Autodesk Inventor part; units mm, degrees
ref_plane "YZ Plane" through (0, 0, 0) normal (1, 0, 0) x (0, 1, 0)
ref_plane "XZ Plane" through (0, 0, 0) normal (0, 1, 0) x (-1, 0, 0)
ref_plane "XY Plane" through (0, 0, 0) normal (0, 0, 1) x (1, 0, 0)
sketch "Sketch1" plane through (0, 0, 0) normal (0, 0, 1) x (1, 0, 0)
  line L0 (0, 12.7112) -> (0, -15.7964)
  line L1 (-14.6857, 0) -> (16.9071, 0)
  line L2 (8.8388, 8.8388) -> (88.8388, -71.1612)
  line L3 (-8.8388, 8.8388) -> (-88.8388, -71.1612)
  line L4 (8.8388, -26.5165) -> (71.1612, -88.8388)
  line L5 (-8.8388, -26.5165) -> (-71.1612, -88.8388)
  arc A0 (8.8388, 8.8388) -> (-8.8388, 8.8388) centre (0, 0) ccw
  arc A1 (8.8388, -26.5165) -> (-8.8388, -26.5165) centre (0, -35.3553) ccw
  arc A2 (71.1612, -88.8388) -> (88.8388, -71.1612) centre (80, -80) ccw
  arc A3 (-88.8388, -71.1612) -> (-71.1612, -88.8388) centre (-80, -80) ccw
  circle A4 centre (-80, -80) radius 3.5
  circle A5 centre (80, -80) radius 3.5
  circle A6 centre (0, 0) radius 8.5
  point P0 (0, 17.6777)
  point P1 (0, -17.6777)
  dimension "d0" = 25
  dimension "d1" = 12.5
  dimension "d2" = 0
  dimension "d3" = 90
  dimension "d4" = 7
  dimension "d5" = 7
  dimension "d8" = 17
  dimension "d17" = 80
extrude "Extrusion1" add sketch "Sketch1" along normal blind 3
sketch "Sketch2" plane through (0, 0, 3) normal (0, 0, 1) x (1, 0, 0)
  circle A0 centre (80, -80) radius 3.5
  line L0 (80, -80) -> (55.28, -55.28)
  line L1 (88.8388, -71.1612) -> (8.8388, 8.8388)
  circle A1 centre (72.0098, -59.6354) radius 1.55
  circle A2 centre (59.6354, -72.0098) radius 1.55
  point P0 (0, 0)
  dimension "d9" = 3.1
  dimension "d10" = 3.1
  dimension "d11" = 21.876
  dimension "d12" = 17.5
extrude "Extrusion2" add sketch "Sketch2" along normal blind 10 contours A1 | A2
mirror "Mirror1" about plane through (0, 0, 0) normal (1, 0, 0) of "Extrusion2"
fillet "Fillet1" radius 2 4 edges at (-70.4598, -59.6354, 3) (-58.0854, -72.0098, 3) (70.4598, -59.6354, 3) (58.0854, -72.0098, 3)
properties part number "rockerbogieçükü"
Check sheet for the modelled part. Datum: model origin and axes. Units: mm. A direction names the side the tool comes from. Round coordinates to 2 decimals unless told otherwise and drop trailing zeros. Loops run counter-clockwise (first coordinate to the right, second up) from the corner with the lowest first, then second, coordinate; pieces in that order, holes last. Notation, with made-up numbers: M 68,-21.5 L 76,-21.5 A29 ccw 76,7.5 Z; hole C 20,27 d7. An arc over 180 degrees is marked long. Answer as a JSON object with one key per item and string values.
1. Section check D-D (y = -13). Record the boundary of the cut face in (x, z).
Reply:
{"outline": "M -30.68,0 L 30.68,0 L 30.68,3 L -30.68,3 Z"}
2. Section check B-B (x = 0). Record the boundary of the cut face in (y, z).
Reply:
{"outline": "M -22.86,0 L -8.5,0 L -8.5,3 L -22.86,3 Z; M 8.5,0 L 12.5,0 L 12.5,3 L 8.5,3 Z"}
3. Access from +Z, -Z, +X, -X, +Y, -Y to the whole of each face (thin tool, end or side, straight path). Record for faces 5 (the flat face through (-39.56, -57.24, 1.48)), 6 (the cylindrical face through (81.615, -76.895, 1.479)).
Reply:
{"face 5": "+Z, -Z, -Y", "face 6": "+Z, -Z"}
4. Scan lines: line 1 (Z direction, x = 13, y = 1); line 2 (Y direction, x = -80, z = 2.25); line 3 (X direction, y = 0, z = 1.55). Record each from-to range of solid material in increasing order.
Reply:
{"line 1": "z = 0 to 3", "line 2": "y = -92.5 to -83.5, -76.5 to -62.32", "line 3": "x = -17.68 to -8.5, 8.5 to 17.68"}
5. Mould release check, pull along Y, two halves, no side actions. Record for faces 1 (the cylindrical face through (4.57, -7.167, 1.479)), 2 (the flat face through (39.56, -57.24, 1.48)), 3 (the cylindrical face through (-78.385, -76.895, 1.479)), 4 (the flat face through (-14, -28, 0)): pulls with the +Y half, pulls with the -Y half, needs draft (parallel to the pull), parting line crosses it, or undercut.
Reply:
{"face 1": "undercut", "face 2": "pulls with the -Y half", "face 3": "undercut", "face 4": "needs draft"}
6. Gauge pin test, flat ends, axial feed: P1, Ø2, axis at x = 13.5, z = 1.5, coming from the +Y side; P2, Ø4, axis at x = -80, y = -80, coming from the -Z side; P3, Ø12, axis at x = -13.5, y = -4, coming from the +Z side; P4, Ø4, axis at y = -1, z = 4.5, coming from the +X side. Record the tip position at first contact, or that the pin passes through.
Reply:
{"P1": "stops at y = 5.18", "P2": "passes through", "P3": "stops at z = 3", "P4": "stops at x = 20"}
7. Section check A-A (y = -35.5). Record the boundary of the cut face in (x, z).
Reply:
{"outline": "M -53.18,0 L -17.82,0 L -17.82,3 L -53.18,3 Z; M 17.82,0 L 53.18,0 L 53.18,3 L 17.82,3 Z"}
8. Section check C-C (z = 8.75). Record the boundary of the cut face in (x, y), plus the area to 3 significant figures.
Reply:
{"outline": "C -72.01,-59.64 d3.1; C -59.64,-72.01 d3.1; C 59.64,-72.01 d3.1; C 72.01,-59.64 d3.1", "area": "30.2 mm²"}
